Here's how the part is built. I have some questions about the finished solid (model axes, mm). A direction names the side the tool comes from. Give positions to 0.01 mm unless a question says otherwise; leave off trailing zeros. Order: outer loops, then holes, each group sorted by start corner. A loop starts at its lowest first (then second) coordinate and runs counter-clockwise, first axis right, second up. Notation, with made-up numbers: M 59,35 L 99,35 A21 cw 99,44 Z; hole C -4.5,80 d2. An arc over 180 degrees is marked long. One line per item, written item: value. Start each with the question number.
from build123d import *

# Parameters (mm, degrees)
SKETCH_1_R          = 7
EXTRUDE_1_DEPTH     = 12
SKETCH_2_R          = 6.4
SKETCH_2_R_2        = 5.6
CUT_EXTRUDE_1_DEPTH = 10
SKETCH_3_R          = 4
EXTRUDE_2_DEPTH     = 14
SKETCH_4_R          = 2
CUT_EXTRUDE_2_DEPTH = 28.820855486
CHAMFER_1_SIZE      = 1.5
CHAMFER_2_SIZE      = 1
FILLET_1_R          = 0.5


with BuildPart() as part:
    # 草图1 → 凸台-拉伸1 (new body)
    with BuildSketch(Plane(origin=(0, 0, 0), x_dir=(0, 0, -1), z_dir=(1, 0, 0))):
        Circle(SKETCH_1_R)
    extrude(amount=EXTRUDE_1_DEPTH)

    # 草图2 → 切除-拉伸1 (cut)
    with BuildSketch(Plane(origin=(12, 0, 0), x_dir=(0, 0, -1), z_dir=(1, 0, 0))):
        Circle(SKETCH_2_R)
        Circle(SKETCH_2_R_2, mode=Mode.SUBTRACT)
    extrude(amount=-CUT_EXTRUDE_1_DEPTH, mode=Mode.SUBTRACT)

    # 草图3 → 凸台-拉伸2 (add)
    with BuildSketch(Plane(origin=(12, 0, 0), x_dir=(0, 0, -1), z_dir=(1, 0, 0))):
        Circle(SKETCH_3_R)
    extrude(amount=EXTRUDE_2_DEPTH)

    # 草图4 → 切除-拉伸2 (cut, through all)
    with BuildSketch(Plane(origin=(26, 0, 0), x_dir=(0, 0, -1), z_dir=(1, 0, 0))):
        Circle(SKETCH_4_R)
    extrude(amount=-CUT_EXTRUDE_2_DEPTH, mode=Mode.SUBTRACT)

    # 倒角1
    chamfer_1_edges = [part.edges().sort_by_distance(p)[0] for p in [
        (0, 0, 2),
    ]]
    chamfer(chamfer_1_edges, length=CHAMFER_1_SIZE)

    # 倒角2
    chamfer_2_edges = [part.edges().sort_by_distance(p)[0] for p in [
        (26, 0, 2),
    ]]
    chamfer(chamfer_2_edges, length=CHAMFER_2_SIZE)

    # 圆角1
    fillet_1_edges = [part.edges().sort_by_distance(p)[0] for p in [
        (26, 0, 4),
        (12, 0, 5.6),
        (12, 0, 6.4),
    ]]
    fillet(fillet_1_edges, radius=FILLET_1_R)


solid = part.part
Item 1: Please list where these lines run through material, in increasing order: probe 1 along Y at (x, z) = (7.25, 0); probe 2 along Y at (x, z) = (19.75, 0); probe 3 along Y at (x, z) = (3.75, -0.5). Write a range as [from, to].
Item 2: For faces 1 (the face through (26, 1, -3)), 2 (the face through (6.816, 0.246, 5.595)), which set-ups out of +Z, -Z, +X, -X, +Y, -Y let a thin tool reach every point of the face, with its end or its side?
Item 3: I want a section at C-C on x = 7.75. Write out the boundary of the cut face in (y, z), plus the area to 3 significant figures.
Item 4: We'd pull the mould along Y, two halves only. Please class faces 3 (the face through (0, -3, -3)), 4 (the face through (18.656, -3.905, 0.867)), 5 (the face through (13, -2, 0)): +Y half, -Y half, draft (parallel to the pull), parting line (faces both ways), or undercut.
Item 5: Will these pins go through, and if not, where does the flat tip stop? P1, Ø4, axis at y = 5, z = -5.5, coming from the +X side; P2, Ø2, axis at x = 11.5, y = -5, coming from the -Z side; P3, Ø1, axis at x = 3, z = -3, coming from the -Y side.
Answer below:
1. probe 1: y = [-7, -6.4], [-5.6, -2], [2, 5.6], [6.4, 7]
1. probe 2: y = [-4, -2], [2, 4]
1. probe 3: y = [-6.98, -6.38], [-5.58, -1.94], [1.94, 5.58], [6.38, 6.98]
2. face 1: +Z, -Z, +X, +Y, -Y
2. face 2: +X
3. outline: C 0,0 d14; C 0,0 d11.2; hole C 0,0 d12.8; hole C 0,0 d4
3. area: 111 mm²
4. face 3: draft
4. face 4: parting line
4. face 5: undercut
5. P1: stops at x = 12
5. P2: stops at z = -5.74
5. P3: stops at y = -6.54
